```python
from build123d import *

# Parameters (mm, degrees)
F1_DEPTH = 52.07
F2_R     = 33.02
F3_R     = 12.7
F4_DEPTH = 27.94
F6_DEPTH = 27.94
F7_R     = 12.7


# Not quite as in the source:
# - a pattern or mirror of a feature is missing from the dataset's text; its kind, count and spacing are read off the source's solid


with BuildPart() as f1:
    # F0 (on Front) → F1 (new body, symmetric)
    with BuildSketch(Plane.XZ):
        with BuildLine():
            Line((-184.15, 27.94), (-184.15, 0))
            Line((-184.15, 0), (-48.26, 0))
            ThreePointArc((-48.26, 0), (-34.1249732601, 34.1249732601), (0, 48.26))
            ThreePointArc((0, 48.26), (34.1249732601, 34.1249732601), (48.26, 0))
            Line((48.26, 0), (184.15, 0))
            Line((184.15, 0), (184.15, 104.14))
            Line((184.15, 104.14), (156.21, 104.14))
            Line((156.21, 104.14), (156.21, 27.94))
            Line((156.21, 27.94), (70.8928515437, 27.94))
            ThreePointArc((70.8928515437, 27.94), (42.880135261, 62.9899515796), (0, 76.2))
            ThreePointArc((0, 76.2), (-42.880135261, 62.9899515796), (-70.8928515437, 27.94))
            Line((-70.8928515437, 27.94), (-184.15, 27.94))
        make_face()
    extrude(amount=F1_DEPTH, both=True)

    # F2
    f2_edges = [f1.edges().sort_by_distance(p)[0] for p in [
        (-184.15, 52.07, 13.97),
        (-184.15, -52.07, 13.97),
    ]]
    fillet(f2_edges, radius=F2_R)

    # F3 (on face) → F4 (cut)
    with BuildSketch(Plane.XY.offset(27.94)):
        with Locations((-151.13, 19.05)):
            Circle(F3_R)
        with Locations((-151.13, -19.05)):
            Circle(F3_R)
    extrude(amount=-F4_DEPTH, mode=Mode.SUBTRACT)

    # F5 (on face) → F6 (cut)
    with BuildSketch(Plane.YZ.offset(184.15)):
        with BuildLine():
            Line((0, 104.14), (0, 55.245))
            ThreePointArc((0, 55.245), (5.8371664787, 57.6628335213), (8.255, 63.5))
            Line((8.255, 63.5), (8.255, 104.14))
            Line((8.255, 104.14), (0, 104.14))
        make_face()
    f6 = extrude(amount=-F6_DEPTH, mode=Mode.SUBTRACT)

    # F6_copies: F6 across plane
    add(f6.mirror(Plane(origin=(0, 0, 0), x_dir=(0, 0, -1), z_dir=(0, -1, 0))), mode=Mode.SUBTRACT)

    # F7
    f7_edges = [f1.edges().sort_by_distance(p)[0] for p in [
        (170.18, -52.07, 104.14),
        (170.18, 52.07, 104.14),
    ]]
    fillet(f7_edges, radius=F7_R)


solid = f1.part
```
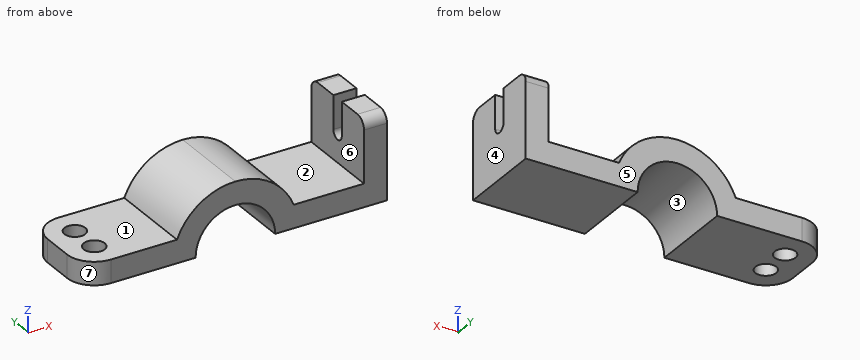
Read the model definition and answer for the solid it produces. Units are mm, in the model's axes. Face numbers are marked on the shaded views. A direction names the side the tool comes from. Coordinates: 2 decimals unless noted, no trailing zeros. Loops run counter-clockwise (first coordinate to the right, second up) from the corner with the lowest first, then second, coordinate; pieces in that order, holes last. Notation, with made-up numbers: (42.5, 61.5) -> (68.5, 61.5) arc R16 cw to (68.5, 73.5) -> close; hole circle Ø8 at (45, 15). An arc over 180 degrees is marked (long way). Return JSON: item names as keys, results as strings.
Item 1: For a pull along X with two mould halves and no side action, classify the marked faces 4, 5, 6 and 7 as +X half, -X half, draft (parallel to the pull), parting line (faces both ways), or undercut.
Answers:
{"face 4": "+X half", "face 5": "draft", "face 6": "undercut", "face 7": "-X half"}
Item 2: Flat-ended cylindrical pins translate along their axes: P1, Ø1, axis at y = -39.5, z = 48.5, coming from the -X side; P2, Ø5, axis at y = -34.5, z = 20.5, coming from the -X side; P3, Ø4, axis at x = 143, y = -29.5, coming from the +Z side; P4, Ø23, axis at x = -151.13, y = 19.05, coming from the -Z side. Find the tip coordinate at first contact, or state that the pin passes through.
Answers:
{"P1": "stops at x = -59.18", "P2": "stops at x = -181.5", "P3": "stops at z = 27.94", "P4": "passes through"}
Item 3: Find the intervals of material crossed by probe 1 along Y at (x, z) = (-151, 19); probe 2 along X at (y, z) = (19, 6); probe 3 along X at (y, z) = (-19, 12), in increasing order.
Answers:
{"probe 1": "y = -52.07 to -31.75, -6.35 to 6.35, 31.75 to 52.07", "probe 2": "x = -184.15 to -163.83, -138.43 to -47.89, 47.89 to 184.15", "probe 3": "x = -184.15 to -163.83, -138.43 to -46.74, 46.74 to 184.15"}
Item 4: Find section A-A (y = 44.5). Determine the outline of the cut face in (x, z), plus the area to 3 significant figures.
Answers:
{"outline": "(-172.17, 0) -> (-48.26, 0) arc R48.26 cw to (48.26, 0) -> (184.15, 0) -> (184.15, 103.06) -> (156.21, 103.06) -> (156.21, 27.94) -> (70.89, 27.94) arc R76.2 ccw to (-70.89, 27.94) -> (-172.17, 27.94) -> close", "area": "13,400 mm2"}
Item 5: For the marked faces 1, 2 and 3, determine the directions among +Z, -Z, +X, -X, +Y, -Y from which every point of the face is accessible in a straight line to the end or side of a thin tool.
Answers:
{"face 1": "+Z, -X, +Y, -Y", "face 2": "+Z, +Y, -Y", "face 3": "-Z, +Y, -Y"}
Item 6: Find section B-B (x = 137.5). Determine the outline of the cut face in (y, z).
Answers:
{"outline": "(-52.07, 0) -> (52.07, 0) -> (52.07, 27.94) -> (-52.07, 27.94) -> close"}
